Job drawing, mm, ordinate dimensions from the low corner. One solid piece. Round coordinates to 2 decimals unless told otherwise and drop trailing zeros. Loops run counter-clockwise (first coordinate to the right, second up) from the corner with the lowest first, then second, coordinate; pieces in that order, holes last. Notation, with made-up numbers: M 79,7 L 103,7 A19 ccw 103,35 Z; hole C 36.5,-29 d7. An arc over 180 degrees is marked long. Put each result on its own line as item: value. Start each with the question number.
1) Slice it at B-B on x = 52. Give the cut face in (y, z).
2) Slice it at A-A on y = 148. Give the cut face in (x, z), then the cut area to 3 significant figures.
3) Drop a flat-ended pin along its axis: pin 1 Ø5 at (x, y) = (155, 121.5) entering from +Z. Give the stop position or say it passes through.
4) Probe line 1 along X through (y, z) = (30, 5.25); line 2 along Z through (x, y) = (136.5, 123.5); line 3 along Z through (x, y) = (3.05, 187). List the from-to ranges inside material, lowest first.
5) Pull direction X, two halves, no side cores. Call the marked faces 1 and 2: +X half, -X half, draft (parallel to the pull), parting line (faces both ways), or undercut.
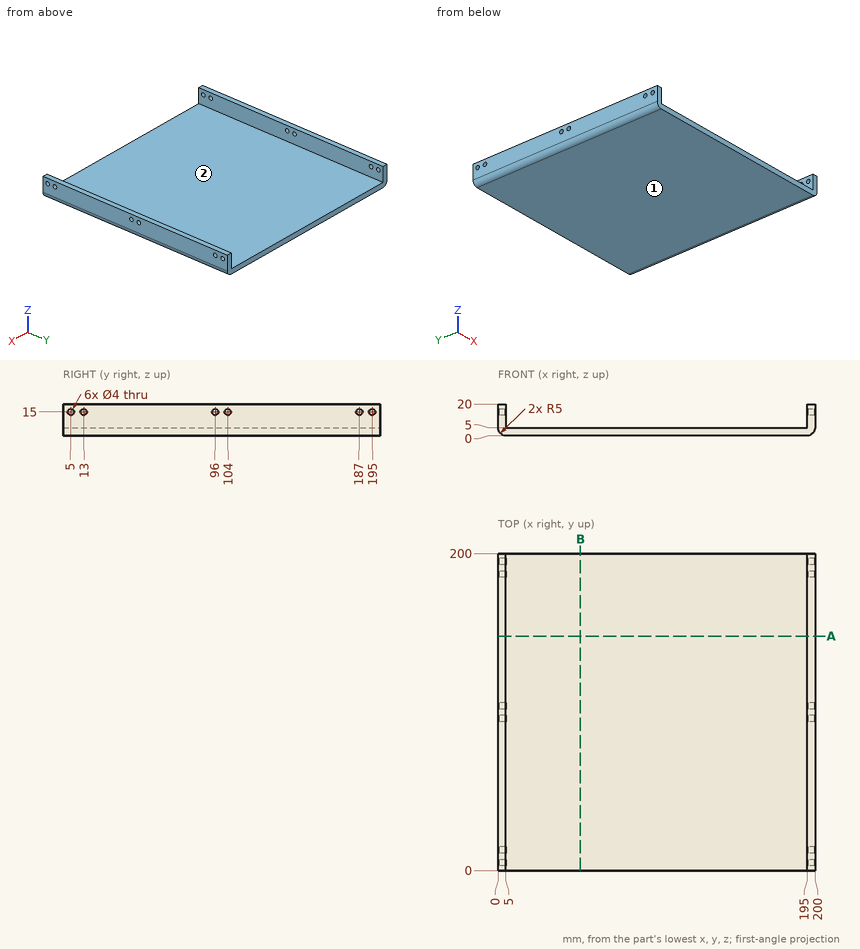
Recorded:
1. outline: M 0,0 L 200,0 L 200,5 L 0,5 Z
2. outline: M 0,5 A5 ccw 5,0 L 195,0 A5 ccw 200,5 L 200,20 L 195,20 L 195,5 L 5,5 L 5,20 L 0,20 Z
2. area: 1,140 mm2
3. pin 1: stops at z = 5
4. line 1: x = 0 to 5, 195 to 200
4. line 2: z = 0 to 5
4. line 3: z = 0.4 to 13, 17 to 20
5. face 1: draft
5. face 2: undercut
